Model file for the job. Use its own axes, mm. A direction names the side the tool comes from. Coordinates: 2 decimals unless noted, no trailing zeros. Write each loop counter-clockwise with the first axis right and the second up, starting at its lowest first coordinate (ties: lowest second). Pieces come first, ordered by that corner, then holes. Notation, with made-up numbers: M 2.25,17 L 49.25,17 A26 cw 49.25,46 Z; hole C 42.5,73.25 d2. An arc over 180 degrees is marked long. Answer in a Markdown table with one row per item. Add a question column.
```python
from build123d import *

# Parameters (mm, degrees)
REVOLVE1_ANGLE     = 180
SKETCH27_R         = 0.75
CUT_EXTRUDE5_DEPTH = 31.850211464
CUT_EXTRUDE6_START = -4
SKETCH27_5_R       = 2.5
SKETCH27_5_R_2     = 0.75
CUT_EXTRUDE6_DEPTH = 10


with BuildPart() as part:
    # Sketch1 → Revolve1 (revolve)
    with BuildSketch(Plane.XY):
        Polygon((6.973429247, -3.10464929), (8.388508538, 5.385826457), (11.829278376, 5.385826457), (11.829278376, 15.385826457), (8.901993981, 15.385826457), (8.640637377, 25.920491769), (4.641867801, 25.8212855), (4.999999973, 11.385826457), (7.829278376, 11.385826457), (7.829278376, 9.385826457), (5.000000185, 9.385826457), (3.027853552, -2.447053341), align=None)
    revolve(axis=Axis((0, 0, 0), (0, 1, 0)), revolution_arc=REVOLVE1_ANGLE)

    # Sketch27 → Cut-Extrude5 (cut, through all)
    with BuildSketch(Plane.XY):
        with Locations((5.965887995, 22.853210278)):
            Circle(SKETCH27_R)
        with Locations((-5.965887995, 22.853210278)):
            Circle(SKETCH27_R)
        with Locations((4.754042918, 0.306629697)):
            Circle(SKETCH27_R)
        with Locations((-4.754042918, 0.306629697)):
            Circle(SKETCH27_R)
    extrude(amount=-CUT_EXTRUDE5_DEPTH, mode=Mode.SUBTRACT)

    # Sketch27<5> → Cut-Extrude6 (cut)
    # profile 1 of 4: a face of its own
    with BuildSketch(Plane.XY.offset(CUT_EXTRUDE6_START)):
        with Locations((5.965887995, 22.853210278)):
            Circle(SKETCH27_5_R)
        with Locations((5.965887995, 22.853210278)):
            Circle(SKETCH27_5_R_2, mode=Mode.SUBTRACT)
    # profile 2 of 4: a face of its own
    with BuildSketch(Plane.XY.offset(CUT_EXTRUDE6_START)):
        with Locations((-5.965887995, 22.853210278)):
            Circle(SKETCH27_5_R)
        with Locations((-5.965887995, 22.853210278)):
            Circle(SKETCH27_5_R_2, mode=Mode.SUBTRACT)
    # profile 3 of 4: a face of its own
    with BuildSketch(Plane.XY.offset(CUT_EXTRUDE6_START)):
        with Locations((4.754042918, 0.306629697)):
            Circle(SKETCH27_5_R)
        with Locations((4.754042918, 0.306629697)):
            Circle(SKETCH27_5_R_2, mode=Mode.SUBTRACT)
    # profile 4 of 4: a face of its own
    with BuildSketch(Plane.XY.offset(CUT_EXTRUDE6_START)):
        with Locations((-4.754042918, 0.306629697)):
            Circle(SKETCH27_5_R)
        with Locations((-4.754042918, 0.306629697)):
            Circle(SKETCH27_5_R_2, mode=Mode.SUBTRACT)
    extrude(amount=-CUT_EXTRUDE6_DEPTH, mode=Mode.SUBTRACT)


solid = part.part
```
1) Which spindle directions (+Z, -Z, +X, -X, +Y, -Y) get a long thin tool onto all of the face, cutting with end or side? Do faces 4 (the face through (0.072, -2.488, -3.274)), 5 (the face through (5.8, 22.12, -1.97)), 6 (the face through (-3.47, 22.7, -5.53)), 7 (the face through (0.1, 3.4, -4)), 8 (the face through (0, 15.386, -10)). Say none if no direction does.
2) Slice it at C-C (z = -0.75). Count the separate pieces of the cut face and the enclosed holes in it, then the cut area to 3 significant figures.
3) Slice it at D-D (y = 6.25). Give the cut face in (x, z), then the cut area to 3 significant figures.
4) Drill centre lines: probe 1 along X at (y, z) = (5.5, -2.75); probe 2 along Y at (x, z) = (-9.5, -3.75); probe 3 along X at (y, z) = (15.25, -1.75). Where is each one in solid material? Low to high.
5) Flat gauge pins, fed straight in: pin 1 Ø3.5 at (x, y) = (-5.5, 0.5) entering from -Z; pin 2 Ø2 at (x, z) = (5.5, -2) entering from +Y; pin 3 Ø1.5 at (x, z) = (5.5, -10) entering from +Y; pin 4 Ø1.2 at (x, y) = (4.75, 0.31) entering from -Z. Where does each tip first touch, or does it go through?
6) Slice it at B-B (x = 0). Give the cut face in (y, z).
7) Two-plate mould, pull along Y, no slides. Class faces 1 (the face through (7, 12, 0)), 2 (the face through (0, 5.386, -9)), 3 (the face through (0.106, 18.503, -4.822)): released by +Y, released by -Y, zero draft, split by the parting line, or undercut.
8) Slice it at A-A (y = 22.5). Give the cut face in (x, z).
Ans:
| question | item | result |
|---|---|---|
| 1 | face 4 | +Z, -Y |
| 1 | face 5 | +Z, -Z |
| 1 | face 6 | -Z |
| 1 | face 7 | +Z |
| 1 | face 8 | -Z, +Y |
| 2 | separate pieces | 2 |
| 2 | enclosed holes | 4 |
| 2 | area | 273 mm2 |
| 3 | outline | M -11.83,0 A11.83 ccw 11.83,0 L 4.48,0 A4.48 cw -4.48,0 Z |
| 3 | area | 188 mm2 |
| 4 | probe 1 | x = -11.51 to -3.37, 3.37 to 11.51 |
| 4 | probe 2 | y = 5.39 to 15.39 |
| 4 | probe 3 | x = -11.7 to -4.58, 4.58 to 11.7 |
| 5 | pin 1 | stops at z = -4 |
| 5 | pin 2 | stops at y = 25.88 |
| 5 | pin 3 | stops at y = 15.39 |
| 5 | pin 4 | passes through |
| 6 | outline | M -3.1,-6.97 L 5.39,-8.39 L 5.39,-11.83 L 15.39,-11.83 L 15.39,-8.9 L 25.92,-8.64 L 25.82,-4.64 L 11.39,-5 L 11.39,-7.83 L 9.39,-7.83 L 9.39,-5 L -2.45,-3.03 Z |
| 7 | face 1 | zero draft |
| 7 | face 2 | released by -Y |
| 7 | face 3 | undercut |
| 8 | outline | M -8.73,0 A8.73 ccw -7.75,-4 L -6.63,-4 L -6.63,0 Z; M -5.3,-4 L -3.49,-4 L -3.49,-8 A8.73 ccw 3.49,-8 L 3.49,-4 L 5.3,-4 L 5.3,0 L 4.72,0 A4.72 cw -4.72,0 L -5.3,0 Z; M 6.63,-4 L 7.75,-4 A8.73 ccw 8.73,0 L 6.63,0 Z |
